Input: part model. Units: mm. Frame: model coordinates. Face numbers are marked on the shaded views. A direction names the side the tool comes from. Coordinates: 2 decimals unless noted, no trailing zeros. Order: outer loops, then holes, each group sorted by start corner. A loop starts at its lowest first (then second) coordinate and runs counter-clockwise, first axis right, second up. Notation, with made-up numbers: (-36.5, 16.5) -> (0.5, 16.5) arc R21 ccw to (0.5, 20.5) -> close; hole circle Ø3 at (1, 14). An arc over 180 degrees is marked (long way). Use one line per item in the form item = value. Start each with the question number.
1) Section query D-D on y = 5. Output: boundary loops of the cut face in (x, z), then the cut area to 3 significant figures.
2) Ray query, line 1 along X through (y, z) = (0, 5.25); line 2 along Y through (x, z) = (0, 17.95); line 3 along Z through (x, y) = (1.75, 0.25). Return the intervals inside material, ascending.
3) Section query C-C on z = 1.75. Output: boundary loops of the cut face in (x, y).
4) Pin query (flat end, axial travel): pin 1 (3.5 mm diameter, centred on x = 0, y = 0, fed in from +Z); pin 2 (2 mm diameter, centred on x = 4, z = 15, fed in from -Y); pin 3 (1.5 mm diameter, centred on y = 1, z = 13.5, fed in from +X). Return the tip coordinate at first contact, or that it passes through.
5) Section query A-A on x = 0. Output: boundary loops of the cut face in (y, z), then the cut area to 3 significant figures.
6) Access query for the marked faces 1 and 2. Directions: +Z, -Z, +X, -X, +Y, -Y. A direction counts if a zero-diameter tool reaches every point of the face in a straight line with its end or side. Return the directions, or none.
7) Section query B-B on y = 0. Output: boundary loops of the cut face in (x, z), then the cut area to 3 significant figures.
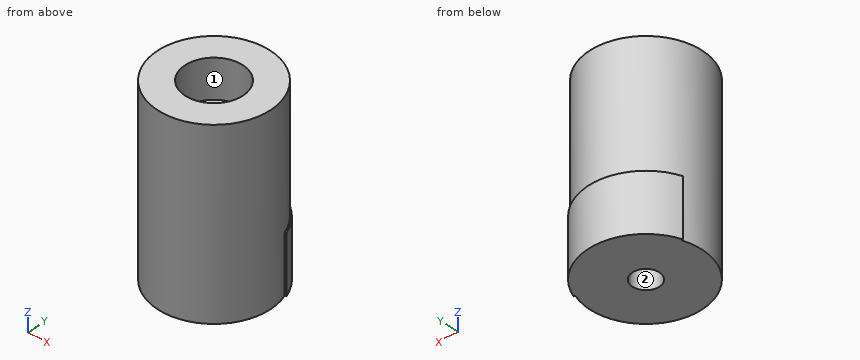
from build123d import *

# Parameters (mm, degrees)
SKETCH011_R     = 5.85
SKETCH011_R_2   = 1.4
PAD002_DEPTH    = 18.9
PAD007_DEPTH    = 6
SKETCH013_R     = 3
POCKET009_DEPTH = 4


with BuildPart() as part:
    # Sketch011 → Pad002 (new body)
    with BuildSketch(Plane.XY):
        Circle(SKETCH011_R)
        Circle(SKETCH011_R_2, mode=Mode.SUBTRACT)
    extrude(amount=PAD002_DEPTH)

    # Sketch012 → Pad007 (join)
    with BuildSketch(Plane.XY):
        with BuildLine():
            ThreePointArc((5.497202, 2.000818), (0, 5.85), (-5.497202, 2.000818))
            Line((-5.497202, 2.000818), (-5.638156, 2.052121))
            ThreePointArc((5.638156, 2.052121), (0, 6), (-5.638156, 2.052121))
            Line((5.497202, 2.000818), (5.638156, 2.052121))
        make_face()
    extrude(amount=PAD007_DEPTH)

    # Sketch013 → Pocket009 (cut)
    with BuildSketch(Plane.XY.offset(18.9)):
        Circle(SKETCH013_R)
    extrude(amount=-POCKET009_DEPTH, mode=Mode.SUBTRACT)


solid = part.part
Answers below:
q1.outline = (-3.32, 0) -> (3.32, 0) -> (3.32, 6) -> (3.04, 6) -> (3.04, 18.9) -> (-3.04, 18.9) -> (-3.04, 6) -> (-3.32, 6) -> close
q1.area = 118 mm^2
q2.line_1 = -5.85 to -1.4, 1.4 to 5.85
q2.line_2 = -5.85 to -3, 3 to 5.85
q2.line_3 = 0 to 14.9
q3.outline = (-5.64, 2.05) -> (-5.5, 2) arc R5.85 ccw (long way) to (5.5, 2) -> (5.64, 2.05) arc R6 ccw to start; hole circle Ø2.8 at (0, 0)
q4.pin_1 = 14.9
q4.pin_2 = -5.02
q4.pin_3 = 5.84
q5.outline = (-5.85, 0) -> (-1.4, 0) -> (-1.4, 14.9) -> (-3, 14.9) -> (-3, 18.9) -> (-5.85, 18.9) -> close; (1.4, 0) -> (6, 0) -> (6, 6) -> (5.85, 6) -> (5.85, 18.9) -> (3, 18.9) -> (3, 14.9) -> (1.4, 14.9) -> close
q5.area = 156 mm^2
q6.face_1 = +Z
q6.face_2 = +Z, -Z
q7.outline = (-5.85, 0) -> (-1.4, 0) -> (-1.4, 14.9) -> (-3, 14.9) -> (-3, 18.9) -> (-5.85, 18.9) -> close; (1.4, 0) -> (5.85, 0) -> (5.85, 18.9) -> (3, 18.9) -> (3, 14.9) -> (1.4, 14.9) -> close
q7.area = 155 mm^2
